Answer from the drawing. Dimensions are ordinates in mm from the lowest x, y and z of the part. A direction names the side the tool comes from. Coordinates: 2 decimals unless noted, no trailing zeros. Loops run counter-clockwise (first coordinate to the right, second up) from the corner with the lowest first, then second, coordinate; pieces in that order, holes last. Notation, with made-up numbers: (-32.75, 25) - (-7.75, 25) arc R20 ccw to (-7.75, 62) - close; hole circle Ø9 at (-38, -23.75). An arc over 180 degrees is marked (long way). Write each question's results on one line, items separated by ' | '. Start each with the question number.
1. A cutting plane is placed at C-C on x = 5. Determine the outline of the cut face in (y, z), then the cut area to 3 significant figures.
2. Which of the six approach directions +Z, -Z, +X, -X, +Y, -Y give full straight-line access (tool end or side, diameter ignored) to the marked faces 1 and 2?
3. Each of these flat-tipped pins is pushed along its axis until it touches: P1, Ø6, axis at x = 36, y = 12.5, coming from the +Z side; P2, Ø6, axis at x = 14, z = 7, coming from the -Y side; P3, Ø6, axis at x = 10, z = 5.5, coming from the +Y side. Where does it stop, or does it pass through?
4. A cutting plane is placed at D-D on x = 35.5. Determine the outline of the cut face in (y, z).
5. Find the intervals of material crossed by line 1 along X through (y, z) = (10.25, 10.25); line 2 along Z through (x, y) = (3, 7.75); line 3 along Y through (x, z) = (10, 8), in increasing order. Write a range as [from, to].
6. A cutting plane is placed at A-A on y = 8. Determine the outline of the cut face in (x, z), then the cut area to 4 significant figures.
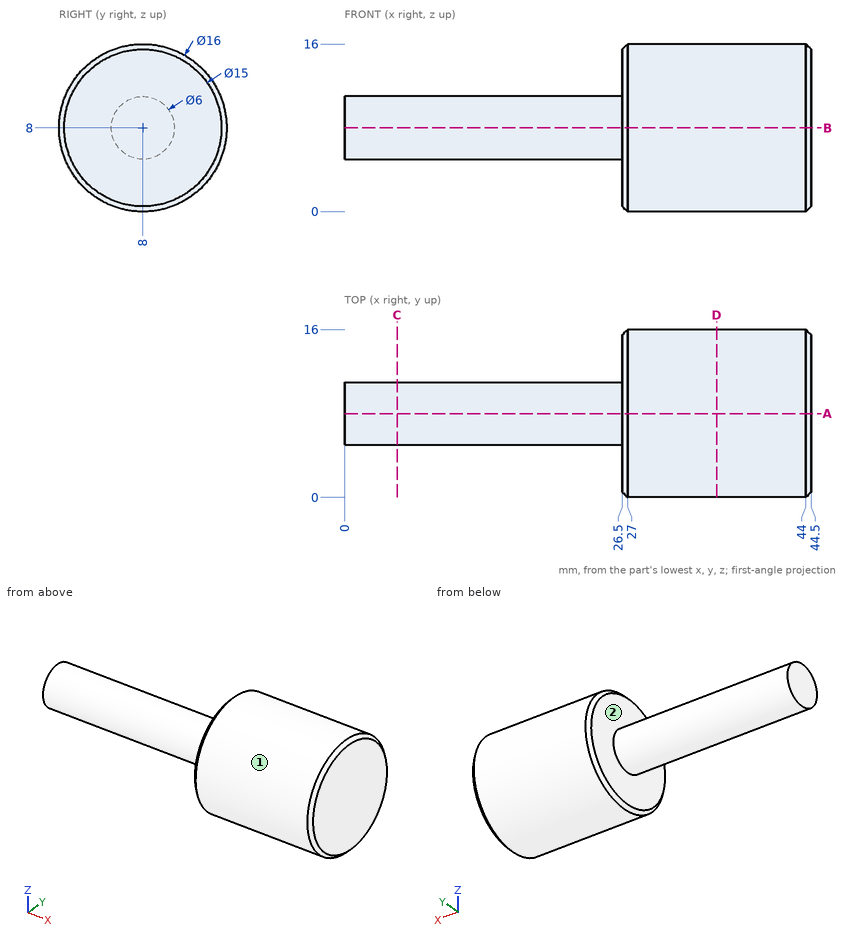
Values:
1) outline: circle Ø6 at (8, 8) | area: 28.3 mm^2
2) face 1: +X, -X | face 2: -X
3) P1: z = 15.86 | P2: y = 5 | P3: y = 11
4) outline: circle Ø16 at (8, 8)
5) line 1: [26.5, 44.5] | line 2: [5.01, 10.99] | line 3: [5, 11]
6) outline: (0, 5) - (26.5, 5) - (26.5, 0.5) - (27, 0) - (44, 0) - (44.5, 0.5) - (44.5, 15.5) - (44, 16) - (27, 16) - (26.5, 15.5) - (26.5, 11) - (0, 11) - close | area: 446.5 mm^2
